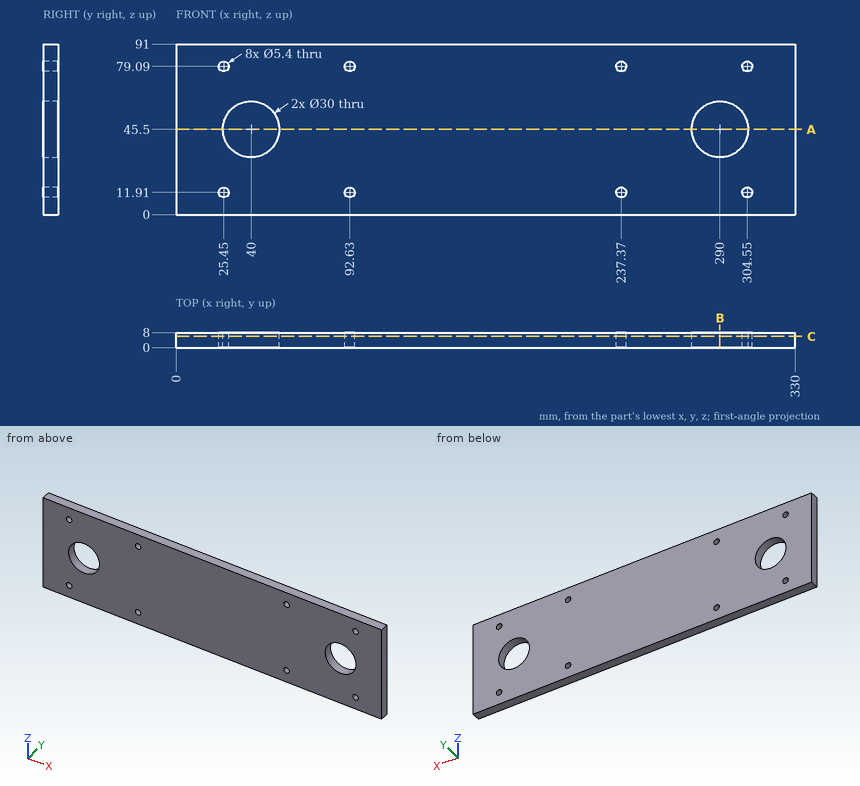
Can you work these out from the drawing? Everything is in mm from the part's minimum corner. Round coordinates to 2 decimals unless told otherwise and drop trailing zeros. Order: outer loops, then holes, each group sorted by start corner. A loop starts at its lowest first (then second) coordinate and runs counter-clockwise, first axis right, second up. Notation, with made-up numbers: (-39.75, -27.75) - (-12.75, -27.75) arc R28 cw to (-12.75, 3.25) - close; hole circle Ø5 at (3.25, 64.5). An arc over 180 degrees is marked (long way). Answer in a Markdown table with one row per item.
(1) Suppose I cut it at A-A, the plane z = 45.5. Please give me the cut outline in (x, y).
From the geometry:
| item | result |
|---|---|
| outline | (0, 0) - (25, 0) - (25, 8) - (0, 8) - close; (55, 0) - (275, 0) - (275, 8) - (55, 8) - close; (305, 0) - (330, 0) - (330, 8) - (305, 8) - close |
(2) Please list where these lines run through material, in increasing order: L1, parallel to Z at x = 92.63, y = 3.75; L2, parallel to X at y = 1.75, z = 45.5; L3, parallel to X at y = 3.5, z = 11.91. Write a range as from..to.
From the geometry:
| item | result |
|---|---|
| L1 | z = 0..9.21, 14.61..76.39, 81.79..91 |
| L2 | x = 0..25, 55..275, 305..330 |
| L3 | x = 0..22.75, 28.15..89.93, 95.33..234.67, 240.07..301.85, 307.25..330 |
(3) Suppose I cut it at B-B, the plane x = 290. Please give me the cut outline in (y, z), plus the area to 3 significant figures.
From the geometry:
| item | result |
|---|---|
| outline | (0, 0) - (8, 0) - (8, 30.5) - (0, 30.5) - close; (0, 60.5) - (8, 60.5) - (8, 91) - (0, 91) - close |
| area | 488 mm2 |
(4) Suppose I cut it at C-C, the plane y = 6. Count the separate pieces of the cut face and the enclosed holes in it, plus the area to 3 significant figures.
From the geometry:
| item | result |
|---|---|
| separate pieces | 1 |
| enclosed holes | 10 |
| area | 28,400 mm2 |
(5) For P1, Ø3, axis at x = 304.55, z = 79.09, coming from the +Y side, with a flat end and sliding along its axis, tell me the tip position at first contact or that it passes through.
From the geometry:
| item | result |
|---|---|
| P1 | passes through |
